Design review of the part built by this model. Coordinates are the model's own, in mm. A direction names the side the tool comes from. Round coordinates to 2 decimals unless told otherwise and drop trailing zeros. Order: outer loops, then holes, each group sorted by start corner. A loop starts at its lowest first (then second) coordinate and runs counter-clockwise, first axis right, second up.
from build123d import *

# Parameters (mm, degrees)
SKETCH_1_R          = 10
SKETCH_1_R_2        = 4
EXTRUDE_1_DEPTH     = 4
SKETCH_2_R          = 7.35
SKETCH_2_R_2        = 3.35
EXTRUDE_2_DEPTH     = 25
SKETCH_3_W          = 15.774529682
SKETCH_3_H          = 4
CUT_EXTRUDE_1_DEPTH = 4


with BuildPart() as part:
    # 草图1 → 拉伸-薄壁1 (new body)
    with BuildSketch(Plane.XY):
        Circle(SKETCH_1_R)
        Circle(SKETCH_1_R_2, mode=Mode.SUBTRACT)
    extrude(amount=EXTRUDE_1_DEPTH)

    # 草图2 → 拉伸-薄壁2 (add)
    with BuildSketch(Plane.XY.offset(4)):
        Circle(SKETCH_2_R)
        Circle(SKETCH_2_R_2, mode=Mode.SUBTRACT)
    extrude(amount=EXTRUDE_2_DEPTH)

    # 草图3 → 切除-拉伸1 (cut)
    with BuildSketch(Plane.XY.offset(29)):
        Rectangle(SKETCH_3_W, SKETCH_3_H)
    extrude(amount=-CUT_EXTRUDE_1_DEPTH, mode=Mode.SUBTRACT)


solid = part.part
1) Take a section at A-A on y = 0. Give the boundary of the cut face in (x, z).
Results:
outline: (-10, 0) - (-4, 0) - (-4, 4) - (-3.35, 4) - (-3.35, 25) - (-7.35, 25) - (-7.35, 4) - (-10, 4) - close; (3.35, 4) - (4, 4) - (4, 0) - (10, 0) - (10, 4) - (7.35, 4) - (7.35, 25) - (3.35, 25) - close
2) To check wall thickness, follow line 1 along Y through (x, z) = (0, 2.35); line 2 along Y through (x, z) = (0, 19). State the ranges of each line that lie inside material, in increasing order.
Results:
line 1: y = -10 to -4, 4 to 10
line 2: y = -7.35 to -3.35, 3.35 to 7.35
3) Take a section at D-D on x = -5.5. Give the boundary of the cut face in (y, z), plus the area to 3 significant figures.
Results:
outline: (-8.35, 0) - (8.35, 0) - (8.35, 4) - (4.88, 4) - (4.88, 29) - (2, 29) - (2, 25) - (-2, 25) - (-2, 29) - (-4.88, 29) - (-4.88, 4) - (-8.35, 4) - close
area: 295 mm2
4) The part is to be moulded in two halves that separate along Y. For faces 5 (the face through (-5, -2, 27)), 6 (the face through (0, -5, 29)), 7 (the face through (-2.17, -9.76, 1.97)), say which applies: released by +Y, released by -Y, zero draft, split by the parting line, or undercut.
Results:
face 5: undercut
face 6: zero draft
face 7: split by the parting line
5) Clearance check with flat-ended pins moving along their axes: P1, Ø1.2, axis at x = 5, z = 27.5, coming from the -Y side; P2, Ø10, axis at x = 3.5, z = 18.5, coming from the +Y side; P3, Ø2, axis at x = 5.5, y = 0, coming from the +Z side; P4, Ø5.5, axis at x = 0, y = 0, coming from the +Z side. State where each tip first meets the part, or that it passes through.
Results:
P1: stops at y = -5.89
P2: stops at y = 7.35
P3: stops at z = 25
P4: passes through
6) Take a section at C-C on z = 17. Give the boundary of the cut face in (x, y).
Results:
outline: circle Ø14.7 at (0, 0); hole circle Ø6.7 at (0, 0)
7) Take a section at B-B on x = 0. Give the boundary of the cut face in (y, z).
Results:
outline: (-10, 0) - (-4, 0) - (-4, 4) - (-3.35, 4) - (-3.35, 29) - (-7.35, 29) - (-7.35, 4) - (-10, 4) - close; (3.35, 4) - (4, 4) - (4, 0) - (10, 0) - (10, 4) - (7.35, 4) - (7.35, 29) - (3.35, 29) - close
8) For faces 1 (the face through (0, 5, 29)), 2 (the face through (0, 7.5, 4)), 3 (the face through (-5, 0, 25)), 4 (the face through (-0.867, -3.905, 1.972)), list the 3-axis set-ups (+Z, -Z, +X, -X, +Y, -Y) from which the entire face can be reached by the end or side of a thin tool; tool diameter is ignored.
Results:
face 1: +Z, +X, -X, +Y, -Y
face 2: +Z
face 3: +Z, +X, -X
face 4: -Z
